Geometry check sheet. Reference: the model listing, model coordinates, mm. A direction names the side the tool comes from. Give positions to 0.01 mm unless a question says otherwise; leave off trailing zeros. Write each loop counter-clockwise with the first axis right and the second up, starting at its lowest first coordinate (ties: lowest second). Pieces come first, ordered by that corner, then holes. Notation, with made-up numbers: (-17, 72.25) - (1, 72.25) arc R36 ccw to (1, 111.25) - close; hole circle Ø1 at (-22, 42.25). An arc over 180 degrees is marked (long way). Write item = value, one per line. Start each with the question number.
(1) Section check A-A, the plane x = -8. Enter the section's corners in (y, z) (3 decimals), plus the area to 3 significant figures.
(2) Access from +Z, -Z, +X, -X, +Y, -Y to the whole of each face (thin tool, end or side, straight path). Record for faces 1 (the flat face through (-19, -9, 72.136)), 2 (the flat face through (-19, 42, 101.6)), 3 (the flat face through (-19, 13, 114.3)), 4 (the flat face through (-2.286, -9, 89)), 5 (the flat face through (-35.814, -9, 89)).
(3) Section check D-D, the plane x = -30. Enter the section's corners in (y, z) (3 decimals), plus the area to 3 significant figures.
(4) Section check C-C, the plane z = 88.9. Enter the section's corners in (x, y) (3 decimals).
(5) Draft check along Y on faces 6 (the flat face through (-38.1, 13, 56)), 7 (the flat face through (-19, 43.18, 89)), 8 (the cylindrical face through (-20.957, 29.47, 82.843)), 9 (the flat face through (-19, 25.4, 56)). Enter one of: pulls with the +Y half, pulls with the -Y half, needs draft (parallel to the pull), parting line crosses it, or undercut.
(6) Thickness scan on L1, parallel to Y at x = -20, z = 109.5 (3 decimals); L2, parallel to Y at x = -10, z = 90.5 (3 decimals); L3, parallel to Y at x = -25.5, z = 24. Record the ranges inside material, lowest first.
(7) Depth check by flat-ended pin: pin 1 Ø12 at (x, z) = (-42, 85.5) entering from +Y (3 decimals); pin 2 Ø15 at (x, y) = (-13, -13.5) entering from -Z; pin 3 Ø1 at (x, y) = (-21.5, 42) entering from +Z. Enter the tip coordinate at first touch or a pass-through.
(8) Section check B-B, the plane z = 110. Enter the section's corners in (x, y) (3 decimals), plus the area to 3 significant figures.
```python
from build123d import *

# Parameters (mm, degrees)
SKETCH1_W           = 38.1
SKETCH1_H           = 25.4
BOSS_EXTRUDE1_DEPTH = 114.3
SKETCH3_W           = 33.528
SKETCH3_H           = 33.528
BOSS_EXTRUDE2_DEPTH = 18.542
SKETCH2_R           = 6.35
BOSS_EXTRUDE3_DEPTH = 17.78
SKETCH4_W           = 25.4
SKETCH4_H           = 25.4
BOSS_EXTRUDE4_DEPTH = 6.35
SKETCH5_R           = 34.1376
BOSS_EXTRUDE5_DEPTH = 3.175


with BuildPart() as part:
    # Sketch1 → Boss-Extrude1 (new body)
    with BuildSketch(Plane.XY):
        with Locations((-19.05, 12.7)):
            Rectangle(SKETCH1_W, SKETCH1_H)
    extrude(amount=BOSS_EXTRUDE1_DEPTH)

    # Sketch3 → Boss-Extrude2 (add)
    with BuildSketch(Plane.XZ):
        with Locations((-19.05, 88.9)):
            Rectangle(SKETCH3_W, SKETCH3_H)
    extrude(amount=BOSS_EXTRUDE2_DEPTH)

    # Sketch2 → Boss-Extrude3 (add)
    with BuildSketch(Plane(origin=(0, 25.4, 0), x_dir=(1, 0, 0), z_dir=(0, 1, 0))):
        with Locations(Location((-19.05, -88.9, 0), (0, 0, 90))):
            Circle(SKETCH2_R)
    extrude(amount=BOSS_EXTRUDE3_DEPTH)

    # Sketch4 → Boss-Extrude4 (add)
    with BuildSketch(Plane(origin=(0, 43.18, 0), x_dir=(1, 0, 0), z_dir=(0, 1, 0))):
        with Locations((-19.05, -88.9)):
            Rectangle(SKETCH4_W, SKETCH4_H)
    extrude(amount=-BOSS_EXTRUDE4_DEPTH)

    # Sketch5 → Boss-Extrude5 (add, symmetric)
    with BuildSketch(Plane.XZ.offset(-36.83)):
        with Locations(Location((-19.450692706, 88.9, 0), (0, 0, 270))):
            Circle(SKETCH5_R)
    extrude(amount=BOSS_EXTRUDE5_DEPTH, both=True)


solid = part.part
```
Model answer:
q1.outline = (-18.542, 72.136) - (0, 72.136) - (0, 0) - (25.4, 0) - (25.4, 114.3) - (0, 114.3) - (0, 105.664) - (-18.542, 105.664) - close; (33.655, 56.74) - (40.005, 56.74) - (40.005, 76.2) - (43.18, 76.2) - (43.18, 101.6) - (40.005, 101.6) - (40.005, 121.06) - (33.655, 121.06) - close
q1.area = 4,010 mm²
q2.face_1 = -Z, +X, -X, -Y
q2.face_2 = +Z, +X, -X, +Y
q2.face_3 = +Z, +X, -X, -Y
q2.face_4 = +Z, -Z, +X, -Y
q2.face_5 = +Z, -Z, -X, -Y
q3.outline = (-18.542, 72.136) - (0, 72.136) - (0, 0) - (25.4, 0) - (25.4, 114.3) - (0, 114.3) - (0, 105.664) - (-18.542, 105.664) - close; (33.655, 56.433) - (40.005, 56.433) - (40.005, 76.2) - (43.18, 76.2) - (43.18, 101.6) - (40.005, 101.6) - (40.005, 121.367) - (33.655, 121.367) - close
q3.area = 4,020 mm²
q4.outline = (-53.588, 33.655) - (-25.4, 33.655) - (-25.4, 25.4) - (-38.1, 25.4) - (-38.1, 0) - (-35.814, 0) - (-35.814, -18.542) - (-2.286, -18.542) - (-2.286, 0) - (0, 0) - (0, 25.4) - (-12.7, 25.4) - (-12.7, 33.655) - (14.687, 33.655) - (14.687, 40.005) - (-6.35, 40.005) - (-6.35, 43.18) - (-31.75, 43.18) - (-31.75, 40.005) - (-53.588, 40.005) - close
q5.face_6 = needs draft
q5.face_7 = pulls with the +Y half
q5.face_8 = undercut
q5.face_9 = undercut
q6.L1 = 0 to 25.4, 33.655 to 40.005
q6.L2 = -18.542 to 25.4, 33.655 to 43.18
q6.L3 = 0 to 25.4
q7.pin_1 = 40.005
q7.pin_2 = 72.14
q7.pin_3 = 101.6
q8.outline = (-46.287, 33.655) - (7.385, 33.655) - (7.385, 40.005) - (-46.287, 40.005) - close; (-38.1, 0) - (0, 0) - (0, 25.4) - (-38.1, 25.4) - close
q8.area = 1,310 mm²
